```python
from build123d import *

# Parameters (mm, degrees)
SKETCH1_W           = 29.4
SKETCH1_H           = 23.1
SKETCH1_R           = 1
BOSS_EXTRUDE1_DEPTH = 2.5
SKETCH2_W           = 29.4
SKETCH2_H           = 2.5
BOSS_EXTRUDE2_DEPTH = 0.5
SKETCH3_W           = 29.4
SKETCH3_H           = 2.5
BOSS_EXTRUDE3_DEPTH = 0.5


with BuildPart() as part:
    # Sketch1 → Boss-Extrude1 (new body)
    with BuildSketch(Plane(origin=(0, 0, 0), x_dir=(1, 0, 0), z_dir=(0, 1, 0))):
        with Locations((-0.8, -0.45)):
            Rectangle(SKETCH1_W, SKETCH1_H)
        with Locations((-9.5, 8.55)):
            Circle(SKETCH1_R, mode=Mode.SUBTRACT)
        with Locations((7.9, 8.55)):
            Circle(SKETCH1_R, mode=Mode.SUBTRACT)
        with Locations((7.9, -9.45)):
            Circle(SKETCH1_R, mode=Mode.SUBTRACT)
        with Locations((-9.5, -9.45)):
            Circle(SKETCH1_R, mode=Mode.SUBTRACT)
    extrude(amount=BOSS_EXTRUDE1_DEPTH)

    # Sketch2 → Boss-Extrude2 (add)
    with BuildSketch(Plane(origin=(0, 0, -11.1), x_dir=(-1, 0, 0), z_dir=(0, 0, -1))):
        with Locations((0.8, 1.25)):
            Rectangle(SKETCH2_W, SKETCH2_H)
    extrude(amount=BOSS_EXTRUDE2_DEPTH)

    # Sketch3 → Boss-Extrude3 (add)
    with BuildSketch(Plane.XY.offset(12)):
        with Locations((-0.8, 1.25)):
            Rectangle(SKETCH3_W, SKETCH3_H)
    extrude(amount=BOSS_EXTRUDE3_DEPTH)


solid = part.part
```
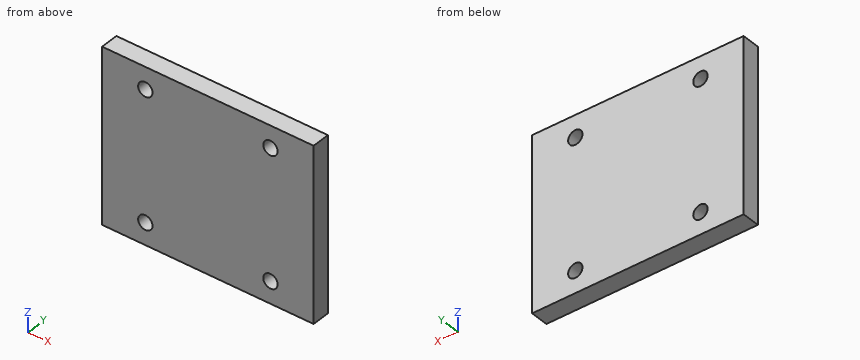
Verification items for the finished model (mm, model axes). Give positions to 0.01 mm unless a question says otherwise; leave off trailing zeros. Order: outer loops, then holes, each group sorted by start corner. A loop starts at its lowest first (then second) coordinate and runs counter-clockwise, first axis right, second up. Notation, with made-up numbers: M 81,29.25 L 108,29.25 A11 ccw 108,34.25 Z; hole C -37.75,-37.75 d3. An arc over 180 degrees is marked long. Return JSON: item names as keys, results as strings. Group by question number.
1) Section check C-C on y = 0.85. Record the cut outline in (x, z), and give its area (3 significant figures).
2) Section check B-B on x = -9.5. Record the cut outline in (y, z).
3) Go/stop test with a flat-tipped pin: pin 1 Ø1.8 at (x, z) = (7.9, 9.45) entering from -Y. Record where the tip stops, or that it passes through.
4) Scan lines: line 1 (X direction, y = 1.3, z = -8.55); line 2 (Z direction, x = -9.5, y = 1.8); line 3 (X direction, y = 2.45, z = -8). Record each from-to range of solid material in increasing order.
5) Section check A-A on z = 9.45. Record the cut outline in (x, y).
Answer block:
{
 "1": {"outline": "M -15.5,-11.6 L 13.9,-11.6 L 13.9,12.5 L -15.5,12.5 Z; hole C -9.5,-8.55 d2; hole C -9.5,9.45 d2; hole C 7.9,-8.55 d2; hole C 7.9,9.45 d2", "area": "696 mm^2"},
 "2": {"outline": "M 0,-11.6 L 2.5,-11.6 L 2.5,-9.55 L 0,-9.55 Z; M 0,-7.55 L 2.5,-7.55 L 2.5,8.45 L 0,8.45 Z; M 0,10.45 L 2.5,10.45 L 2.5,12.5 L 0,12.5 Z"},
 "3": {"pin 1": "passes through"},
 "4": {"line 1": "x = -15.5 to -10.5, -8.5 to 6.9, 8.9 to 13.9", "line 2": "z = -11.6 to -9.55, -7.55 to 8.45, 10.45 to 12.5", "line 3": "x = -15.5 to -10.34, -8.66 to 7.06, 8.74 to 13.9"},
 "5": {"outline": "M -15.5,0 L -10.5,0 L -10.5,2.5 L -15.5,2.5 Z; M -8.5,0 L 6.9,0 L 6.9,2.5 L -8.5,2.5 Z; M 8.9,0 L 13.9,0 L 13.9,2.5 L 8.9,2.5 Z"}
}
